Verification items for the finished model (mm, model axes). Face numbers are marked on the shaded views. A direction names the side the tool comes from. Give positions to 0.01 mm unless a question says otherwise; leave off trailing zeros. Loops run counter-clockwise (first coordinate to the right, second up) from the corner with the lowest first, then second, coordinate; pieces in that order, holes last. Notation, with made-up numbers: M 56,65 L 97,65 A16 ccw 97,83 Z; hole C 45.5,46 d6. An arc over 180 degrees is marked long. Use CSV: the item, a comma, the result in double quotes.
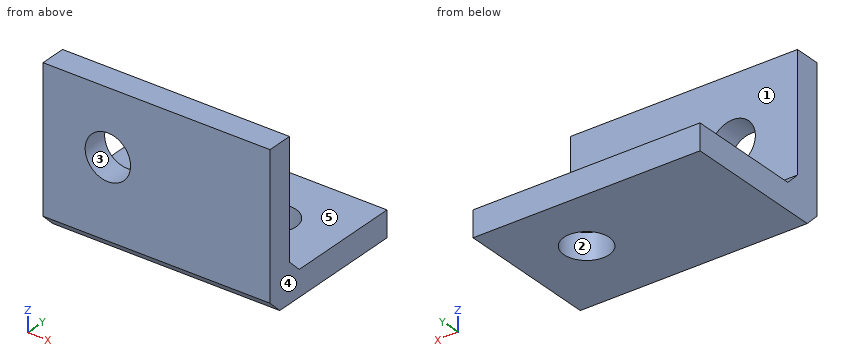
from build123d import *

# Parameters (mm, degrees)
F0_W     = 22.225
F0_H     = 15.24
F0_R     = 2.2225
F1_DEPTH = 2.54
F2_W     = 22.225
F2_H     = 12.7
F2_R     = 2.2225
F3_DEPTH = 2.54
F4_SIZE  = 1.27
F5_SIZE  = 1.27


with BuildPart() as f1:
    # F0 (on Top) → F1 (new body)
    with BuildSketch(Plane.XY):
        with Locations((11.1125, 7.62)):
            Rectangle(F0_W, F0_H)
        with Locations((15.875, 8.89)):
            Circle(F0_R, mode=Mode.SUBTRACT)
    extrude(amount=F1_DEPTH)

    # F2 (on face) → F3 (join)
    with BuildSketch(Plane.XZ):
        with Locations((11.1125, 8.89)):
            Rectangle(F2_W, F2_H)
        with Locations((6.35, 8.89)):
            Circle(F2_R, mode=Mode.SUBTRACT)
    extrude(amount=-F3_DEPTH)

    # F4
    f4_edges = [f1.edges().sort_by_distance(p)[0] for p in [
        (11.1125, 0, 0),
    ]]
    chamfer(f4_edges, length=F4_SIZE)

    # F5
    f5_edges = [f1.edges().sort_by_distance(p)[0] for p in [
        (11.1125, 2.54, 2.54),
    ]]
    chamfer(f5_edges, length=F5_SIZE)


solid = f1.part
(1) Scan lines: L1, parallel to Z at x = 6.35, y = 1.9; L2, parallel to Y at x = 10, z = 10.25. Record each from-to range of solid material in increasing order. Write a range as from..to.
Calculated:
L1,"z = 0..6.67, 11.11..15.24"
L2,"y = 0..2.54"
(2) Depth check by flat-ended pin: pin 1 Ø6 at (x, z) = (6.35, 8.89) entering from +Y; pin 2 Ø1 at (y, z) = (3.5, 11) entering from +X; pin 3 Ø5 at (x, y) = (15.875, 8.89) entering from +Z. Enter the tip coordinate at first touch or a pass-through.
Calculated:
pin 1,"stops at y = 2.54"
pin 2,"passes through"
pin 3,"stops at z = 2.54"
(3) Section check D-D on x = 9.75. Record the cut outline in (y, z), plus the area to 3 significant figures.
Calculated:
outline,"M 0,1.27 L 1.27,0 L 15.24,0 L 15.24,2.54 L 3.81,2.54 L 2.54,3.81 L 2.54,15.24 L 0,15.24 Z"
area,"71.0 mm²"
(4) Section check B-B on x = 6.35. Record the cut outline in (y, z).
Calculated:
outline,"M 0,1.27 L 1.27,0 L 15.24,0 L 15.24,2.54 L 3.81,2.54 L 2.54,3.81 L 2.54,6.67 L 0,6.67 Z; M 0,11.11 L 2.54,11.11 L 2.54,15.24 L 0,15.24 Z"
(5) Section check C-C on z = 8.89. Record the cut outline in (x, y) (1 decimal), plus the area to 3 significant figures.
Calculated:
outline,"M 0,0 L 4.1,0 L 4.1,2.5 L 0,2.5 Z; M 8.6,0 L 22.2,0 L 22.2,2.5 L 8.6,2.5 Z"
area,"45.2 mm²"
(6) Mould release check, pull along Z, two halves, no side actions. Record for the marked faces 3, 4 and 5: released by +Z, released by -Z, zero draft, split by the parting line, or undercut.
Calculated:
face 3,"undercut"
face 4,"zero draft"
face 5,"released by +Z"
(7) Tool access check on the marked faces 1 and 2. Record the directions out of +Z, -Z, +X, -X, +Y, -Y that give a thin tool (end or side, any length) a straight path to the whole face; none if there is none.
Calculated:
face 1,"+Z, +X, -X, +Y"
face 2,"+Z, -Z"
(8) Section check A-A on y = 8.89. Record the cut outline in (x, z) (1 decimal).
Calculated:
outline,"M 0,0 L 13.7,0 L 13.7,2.5 L 0,2.5 Z; M 18.1,0 L 22.2,0 L 22.2,2.5 L 18.1,2.5 Z"
